from build123d import *

# Parameters (mm, degrees)
F2_R    = 3.048
F3_SIZE = 0.762


with BuildPart() as f1:
    # F0 (on Top) → F1 (revolve)
    with BuildSketch(Plane.XY):
        Polygon((-219.829988, 6.35), (-219.829988, 0), (34.170012, 0), (34.170012, 3.175), (27.820012, 3.175), (11.563331, 6.35), align=None)
    revolve(axis=Axis((-92.829988, 0, 0), (-1, 0, 0)))

    # F2
    f2_edges = [f1.edges().sort_by_distance(p)[0] for p in [
        (34.170012, -3.175, 0),
    ]]
    fillet(f2_edges, radius=F2_R)

    # F3
    f3_edges = [f1.edges().sort_by_distance(p)[0] for p in [
        (-219.829988, -6.35, 0),
    ]]
    chamfer(f3_edges, length=F3_SIZE)


solid = f1.part
Source: CAD feature listing. Evaluate the final solid. Frame: model axes, mm. A direction names the side the tool comes from. Coordinates: 2 decimals unless noted, no trailing zeros. Order: outer loops, then holes, each group sorted by start corner. A loop starts at its lowest first (then second) coordinate and runs counter-clockwise, first axis right, second up. Notation, with made-up numbers: M -15.5,-31 L 5.5,-31 A25 cw 5.5,7 Z; hole C -33.5,2.5 d7. An arc over 180 degrees is marked long. Write each question's results on one line, items separated by ' | '. Start each with the question number.
Item 1: Set-up query: faces 1 (the face through (29.45, -0.69, 3.1)), 2 (the face through (-105.37, -1.38, 6.2)). Return all of +Z, -Z, +X, -X, +Y, -Y with unobstructed straight access to the full face (end or side cutting, diameter ignored); none if empty.
Item 2: First-contact query: pin 1 Ø2 at (x, y) = (-50, -4.5) entering from +Z; pin 2 Ø6 at (x, z) = (-46, 2) entering from -Y; pin 3 Ø1 at (x, z) = (-40.5, -4.5) entering from +Y. Flat tips, straight axial feed; report the tip coordinate or a pass-through.
Item 3: Line query: probe 1 along Z at (x, y) = (-208.5, -0.75); probe 2 along Y at (x, z) = (-63.5, 0.5); probe 3 along X at (y, z) = (0, 0.25). Output: solid intervals per line, ascending.
Item 4: Cut plane A-A (x = -13). Return loops of the section in (y, z), and give its area (3 significant figures).
Checked values:
1) face 1: +X | face 2: +X, -X
2) pin 1: stops at z = 5.3 | pin 2: stops at y = -6.35 | pin 3: stops at y = 4.93
3) probe 1: z = -6.31 to 6.31 | probe 2: y = -6.33 to 6.33 | probe 3: x = -219.83 to 34.17
4) outline: C 0,0 d12.7 | area: 127 mm2
